Job drawing, mm, ordinate dimensions from the low corner. One solid piece. A direction names the side the tool comes from. Give positions to 0.01 mm unless a question says otherwise; leave off trailing zeros. Write each loop counter-clockwise with the first axis right and the second up, starting at its lowest first coordinate (ties: lowest second). Pieces come first, ordered by that corner, then holes. Notation, with made-up numbers: M 52,84.25 L 89,84.25 A23 ccw 89,97.25 Z; hole C -18,-7.5 d3. An arc over 180 degrees is marked long. Use a Markdown table: item, result.
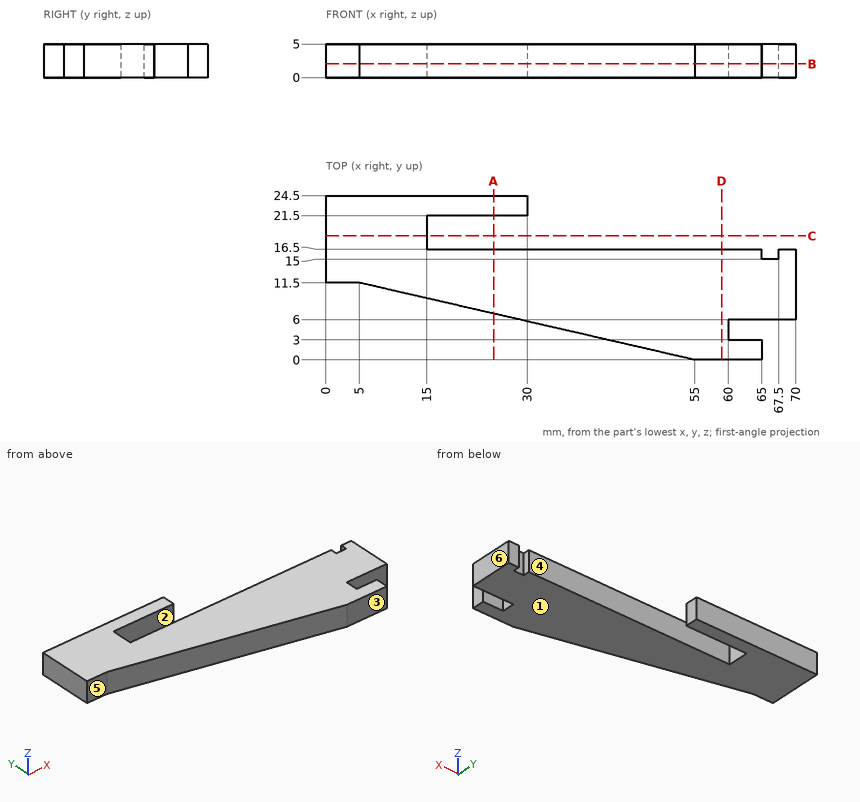
1. Two-plate mould, pull along Y, no slides. Class the marked faces 1, 2 and 3: released by +Y, released by -Y, zero draft, split by the parting line, or undercut.
Findings below:
| item | result |
|---|---|
| face 1 | zero draft |
| face 2 | undercut |
| face 3 | released by -Y |
2. Cut at D-D, the plane x = 59. Give the cut face in (y, z).
Findings below:
| item | result |
|---|---|
| outline | M 0,0 L 16.5,0 L 16.5,5 L 0,5 Z |
3. Cut at B-B, the plane z = 2.05. Give the cut face in (x, y), then the cut area to 3 significant figures.
Findings below:
| item | result |
|---|---|
| outline | M 0,11.5 L 5,11.5 L 55,0 L 65,0 L 65,3 L 60,3 L 60,6 L 70,6 L 70,16.5 L 67.5,16.5 L 67.5,15 L 65,15 L 65,16.5 L 15,16.5 L 15,21.5 L 30,21.5 L 30,24.5 L 0,24.5 Z |
| area | 926 mm2 |
4. Drill centre lines: L1, parallel to X at y = 21.25, z = 0.8; L2, parallel to Y at x = 27.5, z = 0.75 (3 decimals); L3, parallel to Y at x = 27, z = 0.6. Where is each one in solid material? Low to high.
Findings below:
| item | result |
|---|---|
| L1 | 0 to 15 |
| L2 | 6.325 to 16.5, 21.5 to 24.5 |
| L3 | 6.44 to 16.5, 21.5 to 24.5 |
5. Drop flat-ended pins along their axis: P1, Ø1.5, axis at y = 1, z = 3, coming from the +X side; P2, Ø3, axis at x = 66.5, z = 3, coming from the +Y side; P3, Ø1.5, axis at x = 1.5, z = 3.5, coming from the -Y side. Give the stop position or say it passes through.
Findings below:
| item | result |
|---|---|
| P1 | x = 65 |
| P2 | y = 16.5 |
| P3 | y = 11.5 |
6. Cut at C-C, the plane y = 18.5. Give the cut face in (x, z).
Findings below:
| item | result |
|---|---|
| outline | M 0,0 L 15,0 L 15,5 L 0,5 Z |
7. Tool access for the marked faces 4, 5 and 6: list every direction of +Z, -Z, +X, -X, +Y, -Y with a clear straight run to the whole face (end or side of a thin tool).
Findings below:
| item | result |
|---|---|
| face 4 | +Z, -Z, +X |
| face 5 | +Z, -Z, -X, -Y |
| face 6 | +Z, -Z, +X, +Y, -Y |
8. Cut at A-A, the plane x = 25. Give the cut face in (y, z).
Findings below:
| item | result |
|---|---|
| outline | M 6.9,0 L 16.5,0 L 16.5,5 L 6.9,5 Z; M 21.5,0 L 24.5,0 L 24.5,5 L 21.5,5 Z |
